from build123d import *

# Parameters (mm, degrees)
SKETCH_R   = 25
SKETCH_R_2 = 21
SKETCH_R_3 = 19.584537
SKETCH_R_4 = 3
PAD_DEPTH  = 30


with BuildPart() as part:
    # Sketch → Pad (new body)
    with BuildSketch(Plane.XY):
        with BuildLine():
            Line((-81.3335, -100.607731), (84.558204, -100.607731))
            ThreePointArc((84.558204, -100.607731), (97.89969, -95.081507), (103.425914, -81.740021))
            Line((103.425914, -81.740021), (103.425914, 90.030335))
            ThreePointArc((103.425914, 90.030335), (97.36226, 104.66929), (82.723305, 110.732944))
            Line((82.723305, 110.732944), (-80.274155, 110.732944))
            ThreePointArc((-80.274155, 110.732944), (-95.743365, 104.325387), (-102.150922, 88.856177))
            Line((-102.150922, 88.856177), (-102.150922, -79.790309))
            ThreePointArc((-102.150922, -79.790309), (-96.05364, -94.510449), (-81.3335, -100.607731))
        make_face()
        with Locations((0.050005, -0.019529)):
            Circle(SKETCH_R, mode=Mode.SUBTRACT)
        with Locations((-75.610901, -74.830917)):
            Circle(SKETCH_R_2, mode=Mode.SUBTRACT)
        with Locations((77.328041, 85.966019)):
            Circle(SKETCH_R_3, mode=Mode.SUBTRACT)
        with Locations((-35.160095, 24.638546)):
            Circle(SKETCH_R_4, mode=Mode.SUBTRACT)
        with Locations((-35.160095, 5.214603)):
            Circle(SKETCH_R_4, mode=Mode.SUBTRACT)
        with Locations((-55.447323, 5.214603)):
            Circle(SKETCH_R_4, mode=Mode.SUBTRACT)
        with Locations((-76.166206, 4.782958)):
            Circle(SKETCH_R_4, mode=Mode.SUBTRACT)
        with Locations((-55.015682, 44.494133)):
            Circle(SKETCH_R_4, mode=Mode.SUBTRACT)
        with Locations((-0.039441, 29.828697)):
            Circle(SKETCH_R_4, mode=Mode.SUBTRACT)
        with Locations((0.392204, 49.684288)):
            Circle(SKETCH_R_4, mode=Mode.SUBTRACT)
        with Locations((34.150871, 23.956688)):
            Circle(SKETCH_R_4, mode=Mode.SUBTRACT)
        with Locations((54.869728, 44.243923)):
            Circle(SKETCH_R_4, mode=Mode.SUBTRACT)
        with Locations((35.753071, 4.591456)):
            Circle(SKETCH_R_4, mode=Mode.SUBTRACT)
        with Locations((54.74538, 4.591456)):
            Circle(SKETCH_R_4, mode=Mode.SUBTRACT)
        with Locations((75.464256, 4.159811)):
            Circle(SKETCH_R_4, mode=Mode.SUBTRACT)
        with Locations((-34.173149, -15.264144)):
            Circle(SKETCH_R_4, mode=Mode.SUBTRACT)
        with Locations((-54.460381, -35.551373)):
            Circle(SKETCH_R_4, mode=Mode.SUBTRACT)
        with Locations((-0.073334, -30.371653)):
            Circle(SKETCH_R_4, mode=Mode.SUBTRACT)
        with Locations((-0.073334, -50.227249)):
            Circle(SKETCH_R_4, mode=Mode.SUBTRACT)
        with Locations((35.321426, -14.832499)):
            Circle(SKETCH_R_4, mode=Mode.SUBTRACT)
        with Locations((55.177025, -35.983017)):
            Circle(SKETCH_R_4, mode=Mode.SUBTRACT)
    extrude(amount=PAD_DEPTH)


solid = part.part
Geometry check sheet. Reference: the model listing, model coordinates, mm. Give positions to 0.01 mm unless a question says otherwise; leave off trailing zeros. Order: outer loops, then holes, each group sorted by start corner. A loop starts at its lowest first (then second) coordinate and runs counter-clockwise, first axis right, second up. Notation, with made-up numbers: (-6.5, 32.25) - (50.5, 32.25) arc R12 ccw to (50.5, 55.25) - close; hole circle Ø11 at (33.25, 79). An arc over 180 degrees is marked (long way). Use one line per item in the form item = value.
1) Material ranges on probe 1 along Y at (x, z) = (-1.5, 7); probe 2 along Y at (x, z) = (75.5, 9.25); probe 3 along X at (y, z) = (-83.5, 1.75), recorded low to high. Write a range as from..to.
Working result:
probe_1 = -100.61..-52.87, -47.59..-33.01, -27.73..-24.97, 24.93..27.21, 32.45..47.36, 52.01..110.73
probe_2 = -100.61..1.16, 7.16..66.47, 105.47..110.73
probe_3 = -101.82..-94.74, -56.48..103.34
2) Sectioned sample at A-A (y = 93). Record the boundary of the cut face in (x, z), and give its area (3 significant figures).
Working result:
outline = (-101.75, 0) - (59.05, 0) - (59.05, 30) - (-101.75, 30) - close; (95.61, 0) - (103.21, 0) - (103.21, 30) - (95.61, 30) - close
area = 5,050 mm^2
3) Depth check by flat-ended pin: pin 1 Ø5 at (x, y) = (34.15, 23.96) entering from -Z. Enter the tip coordinate at first touch or a pass-through.
Working result:
pin_1 = through
4) Sectioned sample at B-B (z = 15.5). Count the separate pieces of the cut face and the enclosed holes in it, and give its area (3 significant figures).
Working result:
separate_pieces = 1
enclosed_holes = 21
area = 38,000 mm^2
5) Draft check along X on faces 1 (the face through (38.615, 5.493, 14.79)), 2 (the face through (-102.151, 6, 15)), 3 (the face through (22, 30, 0)). Enter one of: released by +X, released by -X, zero draft, split by the parting line, or undercut.
Working result:
face_1 = undercut
face_2 = released by -X
face_3 = zero draft
6) Sectioned sample at C-C (x = 65). Record the boundary of the cut face in (y, z).
Working result:
outline = (-100.61, 0) - (70.75, 0) - (70.75, 30) - (-100.61, 30) - close; (101.18, 0) - (110.73, 0) - (110.73, 30) - (101.18, 30) - close
